Work out the finished part from the listing and answer in its coordinate system (mm). Give positions to 0.01 mm unless a question says otherwise; leave off trailing zeros. One line per item, written item: value.
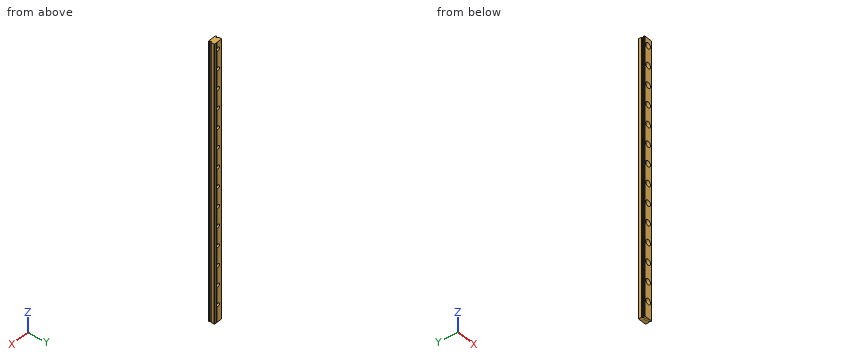
from build123d import *

# Parameters (mm, degrees)
BOSS_EXTRUDE1_START = -144.36216
BOSS_EXTRUDE1_DEPTH = 284.72432
SKETCH2_R           = 1.75
CUT_EXTRUDE1_DEPTH  = 409.901966471
SKETCH2_3_R         = 3
CUT_EXTRUDE2_DEPTH  = 3.5


# Read off the part's stored shape, not the designer's step: Boss-Extrude1
with BuildPart() as part:
    # Boss-Extrude1 outline → Boss-Extrude1 (new body)
    with BuildSketch(Plane.XY.offset(BOSS_EXTRUDE1_START)):
        with BuildLine():
            ThreePointArc((-375.815535559, 396.401159064), (-376.215535559, 396.201159064), (-376.615535559, 396.401159064))
            Line((-376.615535559, 396.401159064), (-382.115535559, 396.401159064))
            Line((-382.115535559, 396.401159064), (-382.515535559, 396.001159064))
            Line((-382.515535559, 396.001159064), (-382.515535559, 392.959462588))
            ThreePointArc((-382.515535559, 392.959462588), (-382.490644208, 392.876710995), (-382.424231211, 392.82142339))
            ThreePointArc((-382.424231211, 392.82142339), (-382.156798336, 392.653535157), (-381.955046042, 392.410630209))
            ThreePointArc((-381.955046042, 392.410630209), (-381.905872585, 392.360101643), (-381.839045976, 392.337621226))
            Line((-381.839045976, 392.337621226), (-381.498104411, 392.307792704))
            ThreePointArc((-381.498104411, 392.307792704), (-381.368080092, 392.243671806), (-381.315535559, 392.108553765))
            Line((-381.315535559, 392.108553765), (-381.315535559, 391.693764363))
            ThreePointArc((-381.315535559, 391.693764363), (-381.368080092, 391.558646322), (-381.498104411, 391.494525424))
            Line((-381.498104411, 391.494525424), (-381.839049723, 391.464696574))
            ThreePointArc((-381.839049723, 391.464696574), (-381.905875926, 391.442216412), (-381.9550493, 391.391688416))
            ThreePointArc((-381.9550493, 391.391688416), (-382.156800742, 391.148786865), (-382.424231211, 390.980900738))
            ThreePointArc((-382.424231211, 390.980900738), (-382.490644208, 390.925613133), (-382.515535559, 390.84286154))
            Line((-382.515535559, 390.84286154), (-382.515535559, 390.301159064))
            Line((-382.515535559, 390.301159064), (-382.115535559, 389.901159064))
            Line((-382.115535559, 389.901159064), (-373.915535559, 389.901159064))
            Line((-373.915535559, 389.901159064), (-373.515535559, 390.301159064))
            Line((-373.515535559, 390.301159064), (-373.515535559, 390.84286154))
            ThreePointArc((-373.515535559, 390.84286154), (-373.540426911, 390.925613132), (-373.606839907, 390.980900738))
            ThreePointArc((-373.606839907, 390.980900738), (-373.874270377, 391.148786865), (-374.076021819, 391.391688416))
            ThreePointArc((-374.076021819, 391.391688416), (-374.125195193, 391.442216412), (-374.192021396, 391.464696574))
            Line((-374.192021396, 391.464696574), (-374.532966708, 391.494525424))
            ThreePointArc((-374.532966708, 391.494525424), (-374.662991027, 391.558646322), (-374.715535559, 391.693764363))
            Line((-374.715535559, 391.693764363), (-374.715535559, 392.108553765))
            ThreePointArc((-374.715535559, 392.108553765), (-374.662991027, 392.243671806), (-374.532966708, 392.307792704))
            Line((-374.532966708, 392.307792704), (-374.192025143, 392.337621226))
            ThreePointArc((-374.192025143, 392.337621226), (-374.125198533, 392.360101643), (-374.076025076, 392.410630209))
            ThreePointArc((-374.076025076, 392.410630209), (-373.874272783, 392.653535157), (-373.606839907, 392.82142339))
            ThreePointArc((-373.606839907, 392.82142339), (-373.540426911, 392.876710996), (-373.515535559, 392.959462588))
            Line((-373.515535559, 392.959462588), (-373.515535559, 396.001159064))
            Line((-373.515535559, 396.001159064), (-373.915535559, 396.401159064))
            Line((-373.915535559, 396.401159064), (-375.815535559, 396.401159064))
        make_face()
    extrude(amount=BOSS_EXTRUDE1_DEPTH)

    # Sketch2 → Cut-Extrude1 (cut, through all)
    with BuildSketch(Plane.XZ.offset(-389.901159064)):
        with Locations(Location((-378.015535559, 132.86216, 0), (0, 0, 270))):
            Circle(SKETCH2_R)
        with Locations(Location((-378.015535559, 112.86216, 0), (0, 0, 270))):
            Circle(SKETCH2_R)
        with Locations(Location((-378.015535559, 92.86216, 0), (0, 0, 270))):
            Circle(SKETCH2_R)
        with Locations(Location((-378.015535559, 72.86216, 0), (0, 0, 270))):
            Circle(SKETCH2_R)
        with Locations(Location((-378.015535559, 52.86216, 0), (0, 0, 270))):
            Circle(SKETCH2_R)
        with Locations(Location((-378.015535559, 32.86216, 0), (0, 0, 270))):
            Circle(SKETCH2_R)
        with Locations(Location((-378.015535559, 12.86216, 0), (0, 0, 270))):
            Circle(SKETCH2_R)
        with Locations(Location((-378.015535559, -7.13784, 0), (0, 0, 270))):
            Circle(SKETCH2_R)
        with Locations(Location((-378.015535559, -27.13784, 0), (0, 0, 270))):
            Circle(SKETCH2_R)
        with Locations(Location((-378.015535559, -47.13784, 0), (0, 0, 270))):
            Circle(SKETCH2_R)
        with Locations(Location((-378.015535559, -67.13784, 0), (0, 0, 270))):
            Circle(SKETCH2_R)
        with Locations(Location((-378.015535559, -87.13784, 0), (0, 0, 270))):
            Circle(SKETCH2_R)
        with Locations(Location((-378.015535559, -107.13784, 0), (0, 0, 270))):
            Circle(SKETCH2_R)
        with Locations(Location((-378.015535559, -127.13784, 0), (0, 0, 270))):
            Circle(SKETCH2_R)
        with Locations((-378.015535559, -147.13784)):
            Circle(SKETCH2_R)
        with Locations((-378.015535559, -167.13784)):
            Circle(SKETCH2_R)
        with Locations((-378.015535559, -187.13784)):
            Circle(SKETCH2_R)
        with Locations((-378.015535559, -207.13784)):
            Circle(SKETCH2_R)
        with Locations((-378.015535559, -227.13784)):
            Circle(SKETCH2_R)
        with Locations((-378.015535559, -247.13784)):
            Circle(SKETCH2_R)
        with Locations((-378.015535559, -267.13784)):
            Circle(SKETCH2_R)
        with Locations((-378.015535559, -287.13784)):
            Circle(SKETCH2_R)
        with Locations((-378.015535559, -307.13784)):
            Circle(SKETCH2_R)
    extrude(amount=-CUT_EXTRUDE1_DEPTH, mode=Mode.SUBTRACT)

    # Sketch2<3> → Cut-Extrude2 (cut)
    with BuildSketch(Plane.XZ.offset(-389.901159064)):
        with Locations(Location((-378.015535559, 132.86216, 0), (0, 0, 270))):
            Circle(SKETCH2_3_R)
        with Locations(Location((-378.015535559, 112.86216, 0), (0, 0, 270))):
            Circle(SKETCH2_3_R)
        with Locations(Location((-378.015535559, 92.86216, 0), (0, 0, 270))):
            Circle(SKETCH2_3_R)
        with Locations(Location((-378.015535559, 72.86216, 0), (0, 0, 270))):
            Circle(SKETCH2_3_R)
        with Locations(Location((-378.015535559, 52.86216, 0), (0, 0, 270))):
            Circle(SKETCH2_3_R)
        with Locations(Location((-378.015535559, 32.86216, 0), (0, 0, 270))):
            Circle(SKETCH2_3_R)
        with Locations(Location((-378.015535559, 12.86216, 0), (0, 0, 270))):
            Circle(SKETCH2_3_R)
        with Locations(Location((-378.015535559, -7.13784, 0), (0, 0, 270))):
            Circle(SKETCH2_3_R)
        with Locations(Location((-378.015535559, -27.13784, 0), (0, 0, 270))):
            Circle(SKETCH2_3_R)
        with Locations(Location((-378.015535559, -47.13784, 0), (0, 0, 270))):
            Circle(SKETCH2_3_R)
        with Locations(Location((-378.015535559, -67.13784, 0), (0, 0, 270))):
            Circle(SKETCH2_3_R)
        with Locations(Location((-378.015535559, -87.13784, 0), (0, 0, 270))):
            Circle(SKETCH2_3_R)
        with Locations(Location((-378.015535559, -107.13784, 0), (0, 0, 270))):
            Circle(SKETCH2_3_R)
        with Locations(Location((-378.015535559, -127.13784, 0), (0, 0, 270))):
            Circle(SKETCH2_3_R)
        with Locations((-378.015535559, -147.13784)):
            Circle(SKETCH2_3_R)
        with Locations((-378.015535559, -167.13784)):
            Circle(SKETCH2_3_R)
    extrude(amount=-CUT_EXTRUDE2_DEPTH, mode=Mode.SUBTRACT)


solid = part.part
(1) Given P1, Ø3, axis at x = -377.5, z = -127, coming from the -Y side; P2, Ø2, axis at x = -378.02, z = -27.14, coming from the +Y side, each flat-ended and moving along its own axis, determine where each tip first touches the part or whether it passes through.
Findings:
P1: stops at y = 393.4
P2: passes through
(2) Find the intervals of material crossed by probe 1 along X at (y, z) = (394.25, 33); probe 2 along Y at (x, z) = (-381.5, -83.5); probe 3 along X at (y, z) = (390.5, -47), in increasing order. Write a range as from..to.
Findings:
probe 1: x = -382.52..-379.76, -376.27..-373.52
probe 2: y = 389.9..391.49, 392.31..396.4
probe 3: x = -382.52..-381.01, -375.02..-373.52
(3) Section A-A, the plane y = 395 is taken. Give the number of separate pieces and of enclosed holes in the cut face, then the cut area to 3 significant figures.
Findings:
separate pieces: 1
enclosed holes: 14
area: 2,430 mm^2
